Geometry: final body of the model. Coordinates: model frame, mm. Give positions to 0.01 mm unless a question says otherwise; leave off trailing zeros. Write each loop counter-clockwise with the first axis right and the second up, starting at its lowest first coordinate (ties: lowest second). Pieces come first, ordered by that corner, then holes. Notation, with made-up numbers: (40.25, -0.5) -> (67.25, -0.5) arc R10 cw to (67.25, 9.5) -> close; hole circle Ø9 at (26, -5.75). An arc over 180 degrees is marked (long way). Answer as a JSON object with one key per item and string values. Group by question number.
(1) Section query B-B on z = 134. Output: boundary loops of the cut face in (x, y).
(2) Material intervals for probe 1 along Y at (x, z) = (54, 136.5), sorted ascending.
(3) Section query A-A on x = -36.5. Output: boundary loops of the cut face in (y, z).
(4) Contact query for flat-ended pins moving along their axis: pin 1 Ø1 at (y, z) = (1, 135) entering from +X; pin 2 Ø12 at (x, z) = (47, 131.5) entering from -Y; pin 3 Ø0.6 at (y, z) = (0.5, 140.5) entering from -X; pin 4 Ø12 at (x, z) = (-25, 127.5) entering from +Y. Output: stop coordinate, or through.
(5) Section query D-D on z = 121. Output: boundary loops of the cut face in (x, y).
(6) Section query C-C on x = -15.5. Output: boundary loops of the cut face in (y, z).
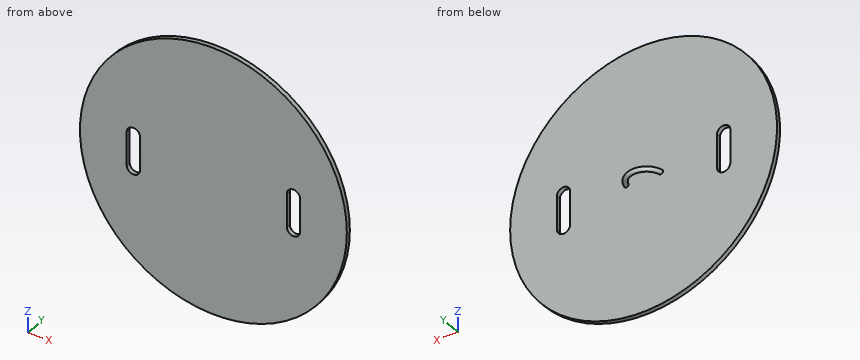
from build123d import *

# Parameters (mm, degrees)
SKETCH1_R           = 60
BOSS_EXTRUDE1_DEPTH = 2
SKETCH3_R           = 1
REVOLVE1_ANGLE      = 180
CUT_EXTRUDE1_DEPTH  = 10


with BuildPart() as part:
    # Sketch1 → Boss-Extrude1 (new body)
    with BuildSketch(Plane(origin=(0, 0, 0), x_dir=(1, 0, 0), z_dir=(0, 1, 0))):
        with Locations((0, -137.725986214)):
            Circle(SKETCH1_R)
    extrude(amount=BOSS_EXTRUDE1_DEPTH)

    # Sketch3 → Revolve1 (revolve)
    with BuildSketch(Plane(origin=(0, 0, 0), x_dir=(1, 0, 0), z_dir=(0, 1, 0))):
        with Locations((8, -137.725986214)):
            Circle(SKETCH3_R)
    revolve(axis=Axis((0, 0, 77.725986214), (0, 0, 1)), revolution_arc=REVOLVE1_ANGLE)

    # Sketch4 → Cut-Extrude1 (cut)
    with BuildSketch(Plane(origin=(0, 2, 0), x_dir=(1, 0, 0), z_dir=(0, 1, 0))):
        with BuildLine():
            Line((39, -129.850097306), (39, -144.850097306))
            ThreePointArc((39, -144.850097306), (36, -147.850097306), (33, -144.850097306))
            Line((33, -144.850097306), (33, -129.850097306))
            ThreePointArc((33, -129.850097306), (36, -126.850097306), (39, -129.850097306))
        make_face()
        with BuildLine():
            Line((-39, -129.850097306), (-39, -144.850097306))
            ThreePointArc((-39, -144.850097306), (-36, -147.850097306), (-33, -144.850097306))
            Line((-33, -144.850097306), (-33, -129.850097306))
            ThreePointArc((-33, -129.850097306), (-36, -126.850097306), (-39, -129.850097306))
        make_face()
    extrude(amount=-CUT_EXTRUDE1_DEPTH, mode=Mode.SUBTRACT)


solid = part.part
Answer list:
{
 "1": {"outline": "(-59.88, 0) -> (-39, 0) -> (-39, 2) -> (-59.88, 2) -> close; (-33, 0) -> (33, 0) -> (33, 2) -> (-33, 2) -> close; (39, 0) -> (59.88, 0) -> (59.88, 2) -> (39, 2) -> close"},
 "2": {"probe 1": "0 to 2"},
 "3": {"outline": "(0, 90.11) -> (2, 90.11) -> (2, 126.89) -> (0, 126.89) -> close; (0, 147.81) -> (2, 147.81) -> (2, 185.35) -> (0, 185.35) -> close"},
 "4": {"pin 1": "x = 59.96", "pin 2": "y = 0", "pin 3": "x = -59.95", "pin 4": "y = 2"},
 "5": {"outline": "(-57.62, 0) -> (57.62, 0) -> (57.62, 2) -> (-57.62, 2) -> close"},
 "6": {"outline": "(0, 79.76) -> (2, 79.76) -> (2, 195.69) -> (0, 195.69) -> close"}
}
